For this review, take the finished solid that the model builds, in its own axes (mm). Face numbers are marked on the shaded views. A direction names the side the tool comes from. Round coordinates to 2 decimals unless told otherwise and drop trailing zeros. Answer in a Markdown table with one row per item.
from build123d import *

# Parameters (mm, degrees)
F0_R     = 30.1625
F0_R_2   = 4.7625
F0_R_3   = 17.4625
F1_DEPTH = 38.1
F2_R     = 30.2476554836
F3_DEPTH = 1.5875


with BuildPart() as f1:
    # F0 (on Top) → F1 (new body)
    with BuildSketch(Plane.XY):
        Circle(F0_R)
        with Locations((-11.90625, -20.6222299276)):
            Circle(F0_R_2, mode=Mode.SUBTRACT)
        with Locations((-20.6222299276, -11.90625)):
            Circle(F0_R_2, mode=Mode.SUBTRACT)
        with Locations((0, -23.8125)):
            Circle(F0_R_2, mode=Mode.SUBTRACT)
        with Locations((11.90625, -20.6222299276)):
            Circle(F0_R_2, mode=Mode.SUBTRACT)
        with Locations((20.6222299276, -11.90625)):
            Circle(F0_R_2, mode=Mode.SUBTRACT)
        with Locations((-23.8125, 0)):
            Circle(F0_R_2, mode=Mode.SUBTRACT)
        with Locations((-20.6222299276, 11.90625)):
            Circle(F0_R_2, mode=Mode.SUBTRACT)
        with Locations((-11.90625, 20.6222299276)):
            Circle(F0_R_2, mode=Mode.SUBTRACT)
        Circle(F0_R_3, mode=Mode.SUBTRACT)
        with Locations((23.8125, 0)):
            Circle(F0_R_2, mode=Mode.SUBTRACT)
        with Locations((20.6222299276, 11.90625)):
            Circle(F0_R_2, mode=Mode.SUBTRACT)
        with Locations((11.90625, 20.6222299276)):
            Circle(F0_R_2, mode=Mode.SUBTRACT)
        with Locations((0, 23.8125)):
            Circle(F0_R_2, mode=Mode.SUBTRACT)
    extrude(amount=F1_DEPTH)

    # F2 (on face) → F3 (join)
    with BuildSketch(Plane(origin=(0, 0, 0), x_dir=(1, 0, 0), z_dir=(0, 0, -1))):
        Circle(F2_R)
    extrude(amount=F3_DEPTH)


solid = f1.part
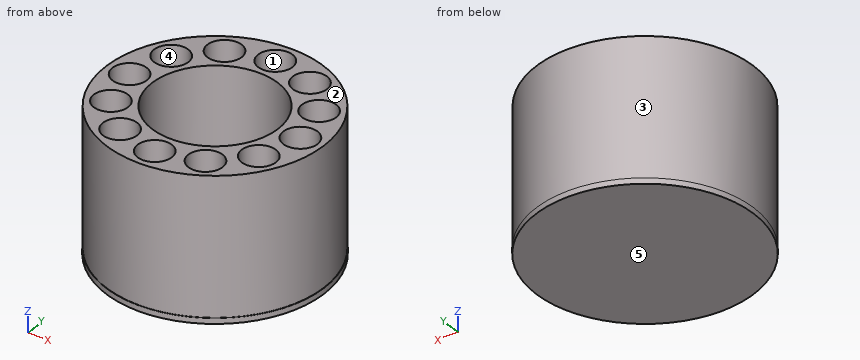
1) For the marked faces 1 and 2, list the 3-axis set-ups (+Z, -Z, +X, -X, +Y, -Y) from which the entire face can be reached by the end or side of a thin tool; tool diameter is ignored.
Solved:
| item | result |
|---|---|
| face 1 | +Z |
| face 2 | +Z, +X, -X, +Y, -Y |
2) For line 1 (X direction, y = -18, z = 33.5); line 2 (Y direction, x = 17.5, z = 27); line 3 (X direction, y = 19, z = 6.5), list the stretches that pass through material, from the lowest coordinate up. Write a range as [from, to].
Solved:
| item | result |
|---|---|
| line 1 | [-24.2, -15.88], [-7.93, 7.93], [15.88, 24.2] |
| line 2 | [-24.57, -15.5], [-8.31, 8.31], [15.5, 24.57] |
| line 3 | [-23.43, -16.38], [-7.43, 7.43], [16.38, 23.43] |
3) Consider section A-A on z = 16.5. State how many separate pieces and enclosed holes the cut face has, then the cut area to 3 significant figures.
Solved:
| item | result |
|---|---|
| separate pieces | 1 |
| enclosed holes | 13 |
| area | 1,050 mm² |
4) Mouldability with a two-part tool opening along Y and no side actions: class the marked faces 3, 4 and 5 as pulls with the +Y half, pulls with the -Y half, needs draft (parallel to the pull), parting line crosses it, or undercut.
Solved:
| item | result |
|---|---|
| face 3 | parting line crosses it |
| face 4 | undercut |
| face 5 | needs draft |
5) Clearance check with flat-ended pins moving along their axes: pin 1 Ø3 at (x, y) = (25, -1) entering from +Z; pin 2 Ø4 at (y, z) = (-21, 9) entering from +X; pin 3 Ø1.5 at (x, z) = (21.5, 18.5) entering from -Y. State where each tip first meets the part, or that it passes through.
Solved:
| item | result |
|---|---|
| pin 1 | z = 0 |
| pin 2 | x = 23.43 |
| pin 3 | y = -21.89 |
